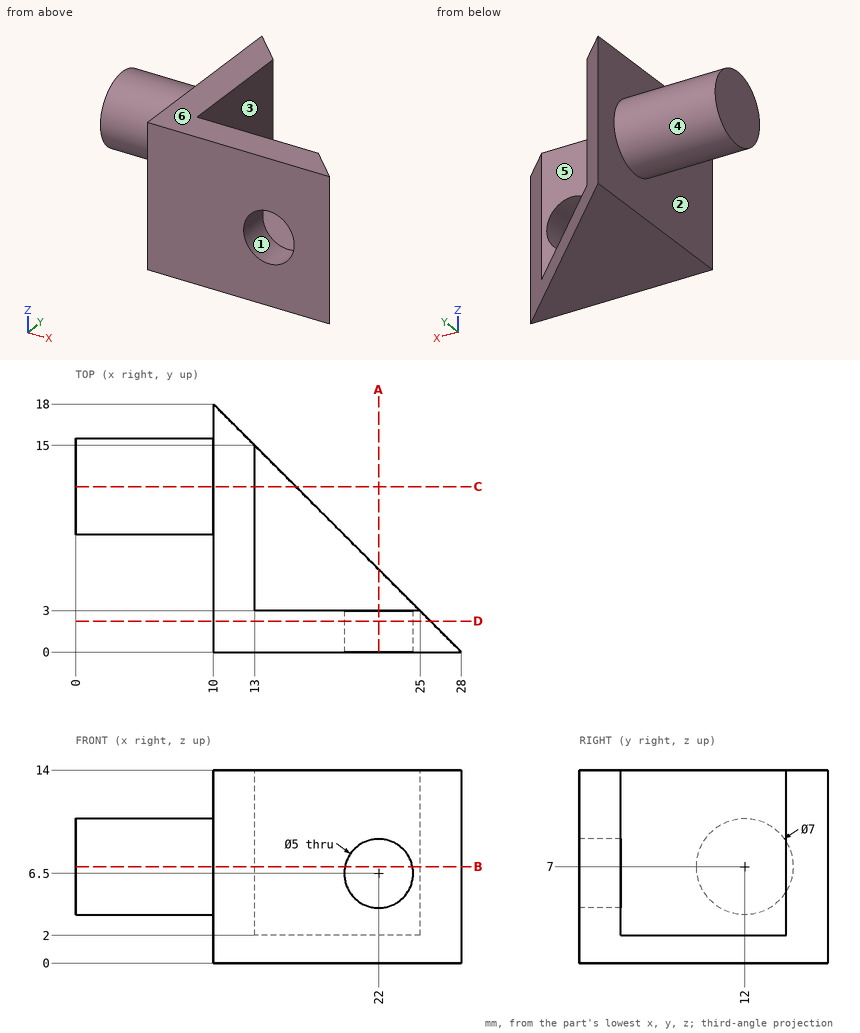
Source: three-view drawing plus pictorial views. Frame: mm from the lowest corner of the part. A direction names the side the tool comes from. Round coordinates to 2 decimals unless told otherwise and drop trailing zeros. Order: outer loops, then holes, each group sorted by start corner. A loop starts at its lowest first (then second) coordinate and runs counter-clockwise, first axis right, second up. Notation, with made-up numbers: (67.5, 7) - (117.5, 7) arc R20 ccw to (117.5, 13) - close; hole circle Ø9 at (42.5, 56.25). An arc over 180 degrees is marked (long way). Answer in a Markdown table with one row per item.
Item 1: Mould query, pull axis X, two halves, no side actions, for the marked faces 1, 2 and 3. Classes: released by +X, released by -X, zero draft, split by the parting line, or undercut.
Model answer:
| item | result |
|---|---|
| face 1 | undercut |
| face 2 | released by -X |
| face 3 | released by +X |
Item 2: Reachability of the marked faces 4, 5 and 6 from +Z, -Z, +X, -X, +Y, -Y: full face, straight path, thin tool, end or side. Return the list, or none.
Model answer:
| item | result |
|---|---|
| face 4 | -X |
| face 5 | +Z, +X, +Y |
| face 6 | +Z, +X, -X, +Y, -Y |
Item 3: Section query A-A (x = 22). Return the cut outline in (y, z), then the cut area to 3 significant figures.
Model answer:
| item | result |
|---|---|
| outline | (0, 0) - (6, 0) - (6, 2) - (3, 2) - (3, 4) - (0, 4) - close; (0, 9) - (3, 9) - (3, 14) - (0, 14) - close |
| area | 33.0 mm² |
Item 4: Section query D-D (y = 2.25). Return the cut outline in (x, z), then the cut area to 3 significant figures.
Model answer:
| item | result |
|---|---|
| outline | (10, 0) - (25.75, 0) - (25.75, 14) - (10, 14) - close; hole circle Ø5 at (22, 6.5) |
| area | 201 mm² |
Item 5: Section query B-B (z = 7). Return the cut outline in (x, y), then the cut area to 3 significant figures.
Model answer:
| item | result |
|---|---|
| outline | (0, 8.5) - (10, 8.5) - (10, 0) - (19.55, 0) - (19.55, 3) - (13, 3) - (13, 15) - (10, 18) - (10, 15.5) - (0, 15.5) - close; (24.45, 0) - (28, 0) - (25, 3) - (24.45, 3) - close |
| area | 145 mm² |
Item 6: Section query C-C (y = 12). Return the cut outline in (x, z).
Model answer:
| item | result |
|---|---|
| outline | (0, 3.5) - (10, 3.5) - (10, 0) - (16, 0) - (16, 2) - (13, 2) - (13, 14) - (10, 14) - (10, 10.5) - (0, 10.5) - close |
Item 7: Line query: line 1 (Z direction, x = 22, y = 0.95); line 2 (Y direction, x = 21.75, z = 11); line 3 (X direction, y = 3.75, z = 9.5). Output: solid intervals per line, ascending.
Model answer:
| item | result |
|---|---|
| line 1 | z = 0 to 4, 9 to 14 |
| line 2 | y = 0 to 3 |
| line 3 | x = 10 to 13 |
Item 8: Pin query (flat end, axial travel): pin 1 (4 mm diameter, centred on y = 6.5, z = 8, fed in from -X); pin 2 (6 mm diameter, centred on y = 10.5, z = 9, fed in from +X); pin 3 (3.5 mm diameter, centred on x = 19, y = 9.5, fed in from +Z); pin 4 (3 mm diameter, centred on x = 22, z = 6.5, fed in from -Y). Return the tip coordinate at first contact, or that it passes through.
Model answer:
| item | result |
|---|---|
| pin 1 | stops at x = 10 |
| pin 2 | stops at x = 13 |
| pin 3 | stops at z = 2 |
| pin 4 | passes through |
